from build123d import *

# Parameters (mm, degrees)
EXTRUDE_1_DEPTH     = 350
CUT_EXTRUDE_1_DEPTH = 360.895818259


with BuildPart() as part:
    # Эскиз1 → Бобышка-Вытянуть1 (new body)
    with BuildSketch(Plane.XY):
        with BuildLine():
            Line((-34, -25), (34, -25))
            ThreePointArc((34, -25), (38.242640687, -23.242640687), (40, -19))
            Line((40, -19), (40, 19))
            ThreePointArc((40, 19), (38.242640687, 23.242640687), (34, 25))
            Line((34, 25), (-34, 25))
            ThreePointArc((-34, 25), (-38.242640687, 23.242640687), (-40, 19))
            Line((-40, 19), (-40, -19))
            ThreePointArc((-40, -19), (-38.242640687, -23.242640687), (-34, -25))
        make_face()
        with BuildLine():
            Line((-34, -21), (34, -21))
            ThreePointArc((34, -21), (35.414213562, -20.414213562), (36, -19))
            Line((36, -19), (36, 19))
            ThreePointArc((36, 19), (35.414213562, 20.414213562), (34, 21))
            Line((34, 21), (-34, 21))
            ThreePointArc((-34, 21), (-35.414213562, 20.414213562), (-36, 19))
            Line((-36, 19), (-36, -19))
            ThreePointArc((-36, -19), (-35.414213562, -20.414213562), (-34, -21))
        make_face(mode=Mode.SUBTRACT)
    extrude(amount=EXTRUDE_1_DEPTH)

    # Эскиз2 → Вырез-Вытянуть1 (cut, through all)
    with BuildSketch(Plane(origin=(40, 0, 0), x_dir=(0, 0, -1), z_dir=(1, 0, 0))):
        with BuildLine():
            Line((-350, 13), (-307, 13))
            ThreePointArc((-307, 13), (-304.878679656, 13.878679656), (-304, 16))
            Line((-304, 16), (-304, 25))
            Line((-304, 25), (-350, 25))
            Line((-350, 25), (-350, 13))
        make_face()
        with BuildLine():
            Line((-181, 13), (-141, 13))
            ThreePointArc((-141, 13), (-138.878679656, 13.878679656), (-138, 16))
            Line((-138, 16), (-138, 25))
            Line((-138, 25), (-184, 25))
            Line((-184, 25), (-184, 16))
            ThreePointArc((-184, 16), (-183.121320344, 13.878679656), (-181, 13))
        make_face()
    extrude(amount=-CUT_EXTRUDE_1_DEPTH, mode=Mode.SUBTRACT)


solid = part.part
Input: part model. Units: mm. Frame: model coordinates. A direction names the side the tool comes from. Coordinates: 2 decimals unless noted, no trailing zeros. Loops run counter-clockwise (first coordinate to the right, second up) from the corner with the lowest first, then second, coordinate; pieces in that order, holes last. Notation, with made-up numbers: (33, 64) - (45, 64) arc R9 cw to (45, 80) - close; hole circle Ø9 at (50, 35). An arc over 180 degrees is marked (long way). Answer in a Markdown table with one row per item. Add a question column.
Item 1: Section query C-C on z = 101.5. Return the cut outline in (x, y).
Item 2: Line query: line 1 along Y through (x, z) = (-12.5, 29.5); line 2 along X through (y, z) = (-2, 206); line 3 along Z through (x, y) = (14, 22). Output: solid intervals per line, ascending. Write a range as [from, to].
Item 3: Mould query, pull axis Y, two halves, no side actions, for faces 4 (the cylindrical face through (38.196, -23.289, 172.55)), 5 (the cylindrical face through (38.289, 23.196, 68.034)), 6 (the flat face through (0, -21, 173)). Classes: released by +Y, released by -Y, zero draft, split by the parting line, or undercut.
Item 4: Section query A-A on x = 26.5. Return the cut outline in (y, z), then the cut area to 3 significant figures.
Item 5: Section query B-B on y = -4.5. Return the cut outline in (x, z).
Item 6: Contact query for flat-ended pins moving along their axis: P1, Ø4.5, axis at x = -16, y = 22, coming from the +Z side; P2, Ø1.2, axis at x = 39, z = 163.5, coming from the +Y side; P3, Ø7, axis at x = 19.5, y = 18.5, coming from the -Z side. Output: stop coordinate, or through.
Item 7: Access query for faces 1 (the flat face through (0, 21, 243)), 2 (the flat face through (1, 22, 304)), 3 (the flat face through (1, 23, 184)). Directions: +Z, -Z, +X, -X, +Y, -Y. A direction counts if a zero-diameter tool reaches every point of the face in a straight line with its end or side. Return the directions, or none.
Recorded:
| question | item | result |
|---|---|---|
| 1 | outline | (-40, -19) arc R6 ccw to (-34, -25) - (34, -25) arc R6 ccw to (40, -19) - (40, 19) arc R6 ccw to (34, 25) - (-34, 25) arc R6 ccw to (-40, 19) - close; hole (-36, -19) arc R2 ccw to (-34, -21) - (34, -21) arc R2 ccw to (36, -19) - (36, 19) arc R2 ccw to (34, 21) - (-34, 21) arc R2 ccw to (-36, 19) - close |
| 2 | line 1 | [-25, -21], [21, 25] |
| 2 | line 2 | [-40, -36], [36, 40] |
| 2 | line 3 | [0, 138], [184, 304] |
| 3 | face 4 | released by -Y |
| 3 | face 5 | released by +Y |
| 3 | face 6 | undercut |
| 4 | outline | (-25, 0) - (-21, 0) - (-21, 350) - (-25, 350) - close; (21, 0) - (25, 0) - (25, 138) - (21, 138) - close; (21, 184) - (25, 184) - (25, 304) - (21, 304) - close |
| 4 | area | 2,430 mm^2 |
| 5 | outline | (-40, 0) - (-36, 0) - (-36, 350) - (-40, 350) - close; (36, 0) - (40, 0) - (40, 350) - (36, 350) - close |
| 6 | P1 | z = 304 |
| 6 | P2 | y = 13 |
| 6 | P3 | z = 0 |
| 7 | face 1 | +Z, -Z |
| 7 | face 2 | +Z, +X, -X, +Y |
| 7 | face 3 | +X, -X, +Y |
